The listing builds one solid part. Answer for the finished solid, in the listing's coordinates (mm). A direction names the side the tool comes from. Round coordinates to 2 decimals unless told otherwise and drop trailing zeros. Loops run counter-clockwise (first coordinate to the right, second up) from the corner with the lowest first, then second, coordinate; pieces in that order, holes last. Notation, with made-up numbers: M -9.75,-24 L 20.25,-24 A32 cw 20.25,2 Z; hole C -29,18.5 d10. An arc over 180 degrees is marked long. Answer as a JSON object with one key per item and string values.
```python
from build123d import *

# Parameters (mm, degrees)
BOSS_EXTRUDE1_DEPTH         = 12.7
SKETCH2_W                   = 11.1252
SKETCH2_H                   = 67.351920908
CUT_EXTRUDE1_DEPTH          = 83.336020747
FILLET1_R                   = 9.525
SKETCH3_R                   = 1.5875
CUT_EXTRUDE2_DEPTH          = 109.624912255
F_1_4_20_TAPPED_HOLE1_D     = 5.1054
F_1_4_20_TAPPED_HOLE2_D     = 5.1054
F_1_4_20_TAPPED_HOLE2_DEPTH = 15.875
F_1_4_20_TAPPED_HOLE2_TIP   = 1.533816902
F_1_4_20_TAPPED_HOLE3_D     = 5.1054


with BuildPart() as part:
    # Sketch1 → Boss-Extrude1 (new, symmetric)
    with BuildSketch(Plane.XY):
        Polygon((-23.8125, -23.8125), (77.7875, -23.8125), (77.7875, 23.8125), (23.8125, 23.8125), align=None)
    boss_extrude1 = extrude(amount=BOSS_EXTRUDE1_DEPTH, both=True)

    # Sketch2 → Cut-Extrude1 (cut, through all)
    with BuildSketch(Plane(origin=(0, 0, 0), x_dir=(0, 0, 1), z_dir=(-0.7071067811865441, 0.707106781186551, 0))):
        Rectangle(SKETCH2_W, SKETCH2_H)
    cut_extrude1 = extrude(amount=-CUT_EXTRUDE1_DEPTH, mode=Mode.SUBTRACT)

    # Mirror1: Boss-Extrude1, Cut-Extrude1 across plane
    add(boss_extrude1.mirror(Plane(origin=(77.7875, 23.8125, 12.7), x_dir=(0, 0, 1), z_dir=(0, -1, 0))))
    add(cut_extrude1.mirror(Plane(origin=(77.7875, 23.8125, 12.7), x_dir=(0, 0, 1), z_dir=(0, -1, 0))), mode=Mode.SUBTRACT)

    # Fillet1
    # the kernel refuses this fillet: 9.525 mm, written as the material it takes off along each edge
    with BuildSketch(Plane(origin=(77.7875, 71.4375, -36.5125), x_dir=(0, -1, 0), z_dir=(0, 0, 1))) as fillet1_piece_1:
        with BuildLine():
            CenterArc((FILLET1_R, -FILLET1_R), FILLET1_R, 90, 90)
            Line((0, -FILLET1_R), (0, 0))
            Line((0, 0), (FILLET1_R, 0))
        make_face()
    extrude(amount=73.025, mode=Mode.SUBTRACT)

    # Sketch3 → Cut-Extrude2 (cut, through all)
    with BuildSketch(Plane.XY.offset(12.7)):
        with Locations((23.8125, 23.8125)):
            Circle(SKETCH3_R)
    extrude(amount=-CUT_EXTRUDE2_DEPTH, mode=Mode.SUBTRACT)

    # 1/4-20 Tapped Hole1 (through all)
    with Locations(Plane.XY.offset(12.7)):
        with Locations((71.4375, 1.5875)):
            Hole(F_1_4_20_TAPPED_HOLE1_D / 2)

    # 1/4-20 Tapped Hole2
    with Locations(Plane(origin=(77.7875, 0, 0), x_dir=(0, 0, -1), z_dir=(1, 0, 0))):
        with Locations((0, 17.4625)):
            Hole(F_1_4_20_TAPPED_HOLE2_D / 2, depth=F_1_4_20_TAPPED_HOLE2_DEPTH)
            with Locations((0, 0, -(F_1_4_20_TAPPED_HOLE2_DEPTH + F_1_4_20_TAPPED_HOLE2_TIP / 2))):  # 118° drill point
                Cone(0, F_1_4_20_TAPPED_HOLE2_D / 2, F_1_4_20_TAPPED_HOLE2_TIP, mode=Mode.SUBTRACT)

    # 1/4-20 Tapped Hole3 (through all)
    with Locations(Plane(origin=(77.7875, 0, 0), x_dir=(0, 0, -1), z_dir=(1, 0, 0))):
        with Locations((0, -14.2875)):
            Hole(F_1_4_20_TAPPED_HOLE3_D / 2)


solid = part.part
```
Item 1: Determine the mould class of faces 1 (the face through (69.739, 19.615, 1.372)), 2 (the face through (23, -3, -5.563)), 3 (the face through (22, 71.438, -9)), 4 (the face through (38, 23, 12.7)) for opening direction Z: released by +Z, released by -Z, zero draft, split by the parting line, or undercut.
Values follow:
{"face 1": "undercut", "face 2": "undercut", "face 3": "zero draft", "face 4": "released by +Z"}
Item 2: The part is cut by section A-A (x = 5). Give the vertices of the cut face in (y, z) (1 decimal).
Values follow:
{"outline": "M -23.8,-12.7 L 5,-12.7 L 5,-5.6 L -23.8,-5.6 Z; M -23.8,5.6 L 5,5.6 L 5,12.7 L -23.8,12.7 Z; M 42.6,-12.7 L 71.4,-12.7 L 71.4,-5.6 L 42.6,-5.6 Z; M 42.6,5.6 L 71.4,5.6 L 71.4,12.7 L 42.6,12.7 Z"}
Item 3: Flat-ended cylindrical pins translate along their axes: P1, Ø1.5, axis at y = 46.5, z = -4.5, coming from the -X side; P2, Ø1, axis at x = -8.5, z = -5, coming from the -Y side; P3, Ø6, axis at y = 5, z = -7.5, coming from the -X side. Find the tip coordinate at first contact, or state that the pin passes through.
Values follow:
{"P1": "x = 45.75", "P2": "through", "P3": "x = 2"}
Item 4: Straight lines are drawn through the part: line 1 (Z direction, x = -1.5, y = 60); line 2 (Y direction, x = 71.25, z = 0) (3 decimals); line 3 (Y direction, x = -3, z = 7.5) (1 decimal). For each, find the intervals that lie inside material, in ascending order.
Values follow:
{"line 1": "-12.7 to -5.56, 5.56 to 12.7", "line 2": "-23.625 to -16.84, -11.735 to -0.958, 4.133 to 14.91, 20.015 to 70.957", "line 3": "-23.8 to -3, 50.6 to 71.4"}
Item 5: The part is cut by section D-D (y = -6). Give the vertices of the cut face in (x, z) (1 decimal).
Values follow:
{"outline": "M -6,-12.7 L 77.8,-12.7 L 77.8,12.7 L -6,12.7 L -6,5.6 L 53.6,5.6 L 53.6,-5.6 L -6,-5.6 Z"}
Item 6: The part is cut by section B-B (y = 51). Give the vertices of the cut face in (x, z) (1 decimal).
Values follow:
{"outline": "M -3.4,-12.7 L 77.8,-12.7 L 77.8,12.7 L -3.4,12.7 L -3.4,5.6 L 51,5.6 L 51,-5.6 L -3.4,-5.6 Z"}
Item 7: The part is cut by section C-C (x = 32). Give the vertices of the cut face in (y, z) (1 decimal), then the cut area to 3 significant figures.
Values follow:
{"outline": "M -23.8,-12.7 L 71.4,-12.7 L 71.4,-5.6 L 32,-5.6 L 32,5.6 L 71.4,5.6 L 71.4,12.7 L -23.8,12.7 L -23.8,5.6 L 15.6,5.6 L 15.6,-5.6 L -23.8,-5.6 Z", "area": "1,540 mm^2"}
Item 8: Which of the six approach directions +Z, -Z, +X, -X, +Y, -Y give full straight-line access (tool end or side, diameter ignored) to faces 5 (the face through (25.4, 23.8, 0.2)), 6 (the face through (48, 48, 0)), 7 (the face through (38, 23, -12.7)), 8 (the face through (48.512, -0.887, 0.078)), 9 (the face through (-0.236, 47.861, -9.081))?
Values follow:
{"face 5": "+Z, -Z", "face 6": "-X, +Y", "face 7": "-Z, +X, -X, +Y, -Y", "face 8": "-X, -Y", "face 9": "+Z, -Z, -X"}
